from build123d import *

# Parameters (mm, degrees)
F0_R     = 2.325
F1_DEPTH = 5.2
F2_R     = 19.035
F2_R_2   = 17.3
F3_DEPTH = 1.48
F6_DEPTH = 49.02
F4_R     = 3.175
F7_DEPTH = 19
F8_W     = 32.18
F8_H     = 7.45
F9_DEPTH = 8.5


with BuildPart() as f1:
    # F0 (on Front) → F1 (new body)
    with BuildSketch(Plane.XZ):
        with BuildLine():
            ThreePointArc((28.1, 23.1), (26.635534, 26.635534), (23.1, 28.1))
            Line((23.1, 28.1), (-23.1, 28.1))
            ThreePointArc((-23.1, 28.1), (-26.635534, 26.635534), (-28.1, 23.1))
            Line((-28.1, 23.1), (-28.1, -23.1))
            ThreePointArc((-28.1, -23.1), (-26.635534, -26.635534), (-23.1, -28.1))
            Line((-23.1, -28.1), (23.1, -28.1))
            ThreePointArc((23.1, -28.1), (26.635534, -26.635534), (28.1, -23.1))
            Line((28.1, -23.1), (28.1, 23.1))
        make_face()
        with Locations((-23.625, -23.625)):
            Circle(F0_R, mode=Mode.SUBTRACT)
        with Locations((23.625, -23.625)):
            Circle(F0_R, mode=Mode.SUBTRACT)
        with Locations((-23.625, 23.625)):
            Circle(F0_R, mode=Mode.SUBTRACT)
        with Locations((23.625, 23.625)):
            Circle(F0_R, mode=Mode.SUBTRACT)
    extrude(amount=F1_DEPTH)

    # F2 (on face) → F3 (join)
    with BuildSketch(Plane.XZ.offset(5.2)):
        Circle(F2_R)
        Circle(F2_R_2, mode=Mode.SUBTRACT)
    extrude(amount=F3_DEPTH)

    # F5 (on face) → F6 (join)
    with BuildSketch(Plane(origin=(0, 0, 0), x_dir=(-1, 0, 0), z_dir=(0, 1, 0))):
        with BuildLine():
            Line((13.7, 28), (-13.7, 28))
            ThreePointArc((-13.7, 28), (-17.235534, 26.535534), (-18.7, 23))
            ThreePointArc((-18.7, 23), (-20.042815, 19.590455), (-23.35, 18.012265))
            ThreePointArc((-23.35, 18.012265), (-26.657185, 16.434076), (-28, 13.02453))
            Line((-28, 13.02453), (-28, -13.02453))
            ThreePointArc((-28, -13.02453), (-26.657185, -16.434076), (-23.35, -18.012265))
            ThreePointArc((-23.35, -18.012265), (-20.042815, -19.590455), (-18.7, -23))
            ThreePointArc((-18.7, -23), (-17.235534, -26.535534), (-13.7, -28))
            Line((-13.7, -28), (13.7, -28))
            ThreePointArc((13.7, -28), (17.235534, -26.535534), (18.7, -23))
            ThreePointArc((18.7, -23), (20.042815, -19.590455), (23.35, -18.012265))
            ThreePointArc((23.35, -18.012265), (26.657185, -16.434076), (28, -13.02453))
            Line((28, -13.02453), (28, 13.02453))
            ThreePointArc((28, 13.02453), (26.657185, 16.434076), (23.35, 18.012265))
            ThreePointArc((23.35, 18.012265), (20.042815, 19.590455), (18.7, 23))
            ThreePointArc((18.7, 23), (17.235534, 26.535534), (13.7, 28))
        make_face()
    extrude(amount=F6_DEPTH)

    # F4 (on face) → F7 (join)
    with BuildSketch(Plane.XZ.offset(5.2)):
        Circle(F4_R)
    extrude(amount=F7_DEPTH)

    # F8 (on face) → F9 (join, symmetric)
    with BuildSketch(Plane(origin=(0, 0, -28), x_dir=(1, 0, 0), z_dir=(0, 0, -1))):
        with Locations((0, -40.405)):
            Rectangle(F8_W, F8_H)
    extrude(amount=F9_DEPTH, both=True)


solid = f1.part
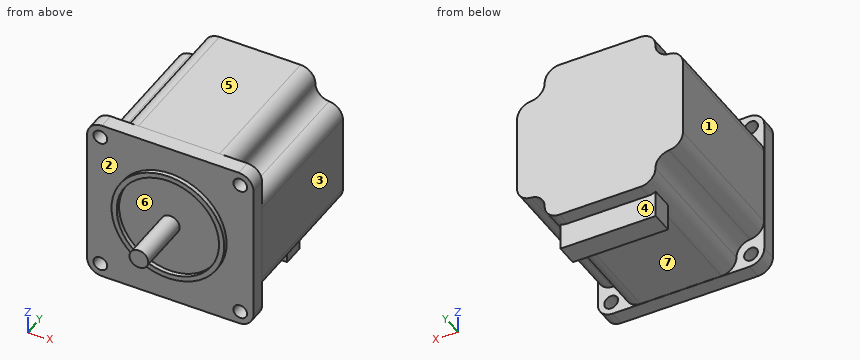
Verification items for the finished model (mm, model axes). Face numbers are marked on the shaded views. A direction names the side the tool comes from. Coordinates: 2 decimals unless noted, no trailing zeros. Order: outer loops, then holes, each group sorted by start corner. A loop starts at its lowest first (then second) coordinate and runs counter-clockwise, first axis right, second up. Notation, with made-up numbers: M 21.25,81.5 L 42.25,81.5 A10 ccw 42.25,88.5 Z; hole C -12.5,42 d9. An arc over 180 degrees is marked long. Write each question's results on one line, items separated by ' | '.
1) Section check B-B on y = 42. Record the cut outline in (x, z).
Solved:
outline: M -28,-13.02 A5 ccw -23.35,-18.01 A5 cw -18.7,-23 A5 ccw -16.09,-27.39 L -16.09,-36.5 L 16.09,-36.5 L 16.09,-27.39 A5 ccw 18.7,-23 A5 cw 23.35,-18.01 A5 ccw 28,-13.02 L 28,13.02 A5 ccw 23.35,18.01 A5 cw 18.7,23 A5 ccw 13.7,28 L -13.7,28 A5 ccw -18.7,23 A5 cw -23.35,18.01 A5 ccw -28,13.02 Z
2) Section check C-C on x = 0. Record the cut outline in (y, z) (3 decimals).
Solved:
outline: M -24.2,-3.175 L -5.2,-3.175 L -5.2,-17.3 L -6.68,-17.3 L -6.68,-19.035 L -5.2,-19.035 L -5.2,-28.1 L 0,-28.1 L 0,-28 L 36.68,-28 L 36.68,-36.5 L 44.13,-36.5 L 44.13,-28 L 49.02,-28 L 49.02,28 L 0,28 L 0,28.1 L -5.2,28.1 L -5.2,19.035 L -6.68,19.035 L -6.68,17.3 L -5.2,17.3 L -5.2,3.175 L -24.2,3.175 Z
3) Release check for a two-part mould opening along Z. For the marked faces 4, 5, 6 and 7 record: pulls with the +Z half, pulls with the -Z half, needs draft (parallel to the pull), parting line crosses it, or undercut.
Solved:
face 4: needs draft | face 5: pulls with the +Z half | face 6: undercut | face 7: pulls with the -Z half
4) Access from +Z, -Z, +X, -X, +Y, -Y to the whole of each face (thin tool, end or side, straight path). Record for the marked faces 1, 2 and 3.
Solved:
face 1: +Z, -Z, -X, +Y | face 2: -Y | face 3: +Z, -Z, +X, +Y
5) Section check A-A on z = 0. Record the cut outline in (x, y) (3 decimals).
Solved:
outline: M -28.1,-5.2 L -19.035,-5.2 L -19.035,-6.68 L -17.3,-6.68 L -17.3,-5.2 L -3.175,-5.2 L -3.175,-24.2 L 3.175,-24.2 L 3.175,-5.2 L 17.3,-5.2 L 17.3,-6.68 L 19.035,-6.68 L 19.035,-5.2 L 28.1,-5.2 L 28.1,0 L 28,0 L 28,49.02 L -28,49.02 L -28,0 L -28.1,0 Z
6) Scan lines: line 1 along Z through (x, y) = (0, -5.7) (3 decimals); line 2 along Y through (x, z) = (-19.5, 6); line 3 along Z through (x, y) = (-12, 39). Record each from-to range of solid material in increasing order. Write a range as [from, to].
Solved:
line 1: z = [-19.035, -17.3], [-3.175, 3.175], [17.3, 19.035] | line 2: y = [-5.2, 49.02] | line 3: z = [-36.5, 28]
7) Gauge pin test, flat ends, axial feed: pin 1 Ø3 at (x, z) = (-23.625, 23.625) entering from +Y; pin 2 Ø1.5 at (x, z) = (19.5, 13.5) entering from -Y; pin 3 Ø7.5 at (x, z) = (-23.625, -23.625) entering from +Y; pin 4 Ø1.5 at (x, y) = (-1, 47) entering from -Z. Record the tip position at first contact, or that the pin passes through.
Solved:
pin 1: passes through | pin 2: stops at y = -5.2 | pin 3: stops at y = 0 | pin 4: stops at z = -28
8) Section check D-D on x = 7. Record the cut outline in (y, z).
Solved:
outline: M -6.68,-17.7 L -5.2,-17.7 L -5.2,-28.1 L 0,-28.1 L 0,-28 L 36.68,-28 L 36.68,-36.5 L 44.13,-36.5 L 44.13,-28 L 49.02,-28 L 49.02,28 L 0,28 L 0,28.1 L -5.2,28.1 L -5.2,17.7 L -6.68,17.7 L -6.68,15.82 L -5.2,15.82 L -5.2,-15.82 L -6.68,-15.82 Z
